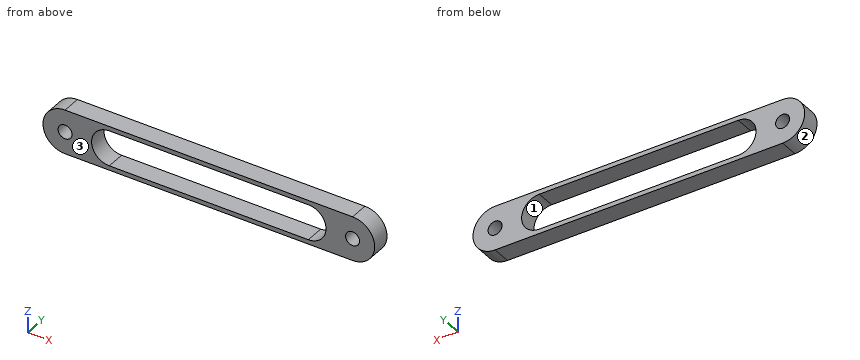
from build123d import *

# Parameters (mm, degrees)
BOSS_EXTRU_1_DEPTH      = 4.25
ESQUISSE2_R             = 3.15
ENL_V_MAT_EXTRU_1_DEPTH = 9.5


with BuildPart() as part:
    # Esquisse1 → Boss.-Extru.1 (new body, symmetric)
    with BuildSketch(Plane(origin=(0, 0, 0), x_dir=(1, 0, 0), z_dir=(0, 1, 0))):
        with BuildLine():
            Line((0, 10), (130, 10))
            ThreePointArc((130, 10), (140, 0), (130, -10))
            Line((130, -10), (0, -10))
            ThreePointArc((0, -10), (-10, 0), (0, 10))
        make_face()
        with BuildLine():
            Line((20, 8), (110, 8))
            ThreePointArc((110, 8), (118, 0), (110, -8))
            Line((110, -8), (20, -8))
            ThreePointArc((20, -8), (12, 0), (20, 8))
        make_face(mode=Mode.SUBTRACT)
    extrude(amount=BOSS_EXTRU_1_DEPTH, both=True)

    # Esquisse2 → Enlèv. mat.-Extru.1 (cut, through all)
    with BuildSketch(Plane(origin=(0, 4.25, 0), x_dir=(1, 0, 0), z_dir=(0, 1, 0))):
        Circle(ESQUISSE2_R)
        with Locations((130, 0)):
            Circle(ESQUISSE2_R)
    extrude(amount=-ENL_V_MAT_EXTRU_1_DEPTH, mode=Mode.SUBTRACT)


solid = part.part
Input: part model. Units: mm. Frame: model coordinates. Face numbers are marked on the shaded views. Coordinates: 2 decimals unless noted, no trailing zeros. Order: outer loops, then holes, each group sorted by start corner. A loop starts at its lowest first (then second) coordinate and runs counter-clockwise, first axis right, second up. Notation, with made-up numbers: M 13.25,16 L 32.25,16 A25 cw 32.25,45 Z; hole C 59,14.25 d9. An arc over 180 degrees is marked long. One line per question, with ' | ' between items.
Item 1: Section C-C (y = -1). Output: boundary loops of the cut face in (x, z), then the cut area to 3 significant figures.
Geometry results:
outline: M 0,-10 L 130,-10 A10 ccw 130,10 L 0,10 A10 ccw Z; hole C 0,0 d6.3; hole M 20,-8 L 110,-8 A8 ccw 110,8 L 20,8 A8 ccw Z; hole C 130,0 d6.3 | area: 1,210 mm^2
Item 2: Draft query along Z for the marked faces 1, 2 and 3. Return one class per face: released by +Z, released by -Z, zero draft, split by the parting line, or undercut.
Geometry results:
face 1: undercut | face 2: split by the parting line | face 3: zero draft
Item 3: Section B-B (z = 0). Output: boundary loops of the cut face in (x, y).
Geometry results:
outline: M -10,-4.25 L -3.15,-4.25 L -3.15,4.25 L -10,4.25 Z; M 3.15,-4.25 L 12,-4.25 L 12,4.25 L 3.15,4.25 Z; M 118,-4.25 L 126.85,-4.25 L 126.85,4.25 L 118,4.25 Z; M 133.15,-4.25 L 140,-4.25 L 140,4.25 L 133.15,4.25 Z
Item 4: Pin query (flat end, axial travel): pin 1 (1.5 mm diameter, centred on y = 3, z = -1, fed in from -X); pin 2 (2 mm diameter, centred on y = 1, z = 6, fed in from -X). Return the tip coordinate at first contact, or that it passes through.
Geometry results:
pin 1: stops at x = -10 | pin 2: stops at x = -8.66
Item 5: Section A-A (x = 100.5). Output: boundary loops of the cut face in (y, z), then the cut area to 3 significant figures.
Geometry results:
outline: M -4.25,-10 L 4.25,-10 L 4.25,-8 L -4.25,-8 Z; M -4.25,8 L 4.25,8 L 4.25,10 L -4.25,10 Z | area: 34.0 mm^2
Item 6: Ray query, line 1 along X through (y, z) = (-1.25, 0); line 2 along Z through (x, y) = (45, 0); line 3 along Z through (x, y) = (0, 1.25). Return the intervals inside material, ascending.
Geometry results:
line 1: x = -10 to -3.15, 3.15 to 12, 118 to 126.85, 133.15 to 140 | line 2: z = -10 to -8, 8 to 10 | line 3: z = -10 to -3.15, 3.15 to 10
